Read the model definition and answer for the solid it produces. Units are mm, in the model's axes. Face numbers are marked on the shaded views. A direction names the side the tool comes from. Round coordinates to 2 decimals unless told otherwise and drop trailing zeros. Loops run counter-clockwise (first coordinate to the right, second up) from the corner with the lowest first, then second, coordinate; pieces in that order, holes last. Notation, with made-up numbers: (12.5, 52) - (69.5, 52) arc R21 ccw to (69.5, 80) - close; hole circle Ø10 at (-35.75, 87.25). An arc over 180 degrees is marked (long way). Answer as CSV lines item,"result".
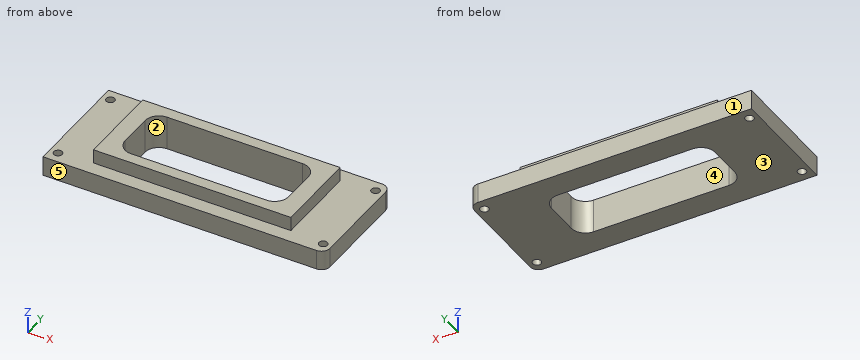
Solid Edge part; units mm, degrees
sketch "Sketch1" plane through (0, 0, 0) normal (0, 0, 1) x (1, 0, 0)
  line L0 (13.4496, 3.5507) -> (113.4496, 3.5507)
  line L1 (113.4496, 3.5507) -> (113.4496, 43.5507)
  line L2 (113.4496, 43.5507) -> (13.4496, 43.5507)
  line L3 (13.4496, 43.5507) -> (13.4496, 3.5507)
extrude "Protrusion1" add sketch "Sketch1" along normal blind 7
hole "Hole_1" at (16.4496, 39.5507, 7) direction (0, 0, -1) diameter 3 end through all
hole "Hole1" at (16.4496, 7.5507, 7) direction (0, 0, -1) diameter 3 end through all
hole "Hole2" at (110.4496, 7.5507, 7) direction (0, 0, -1) diameter 3 end through all
hole "Hole3" at (110.4496, 39.5507, 7) direction (0, 0, -1) diameter 3 end through all
sketch "Sketch2" plane through (63.4496, 23.5507, 7) normal (0, 0, 1) x (1, 0, 0)
  line L0 (-35, 15) -> (35, 15)
  line L1 (35, 15) -> (35, -15)
  line L2 (35, -15) -> (-35, -15)
  line L3 (-35, -15) -> (-35, 15)
extrude "ExtrudedProtrusion_2" add sketch "Sketch2" along normal blind 5
sketch "Sketch3" plane through (63.4496, 23.5507, 12) normal (0, 0, 1) x (0, 1, 0)
  line L0 (-11, -29) -> (11, -29)
  line L1 (11, -29) -> (11, 29)
  line L2 (11, 29) -> (-11, 29)
  line L3 (-11, 29) -> (-11, -29)
  dimension "D1" = 11
  dimension "D2" = 11
extrude "Cutout1" cut sketch "Sketch3" against normal through all
fillet "Round_2" radius 5 4 edges at (34.4496, 34.5507, 6) (34.4496, 12.5507, 6) (92.4496, 12.5507, 6) (92.4496, 34.5507, 6)
fillet "Round_4" radius 3 2 edges at (113.4496, 43.5507, 3.5) (113.4496, 3.5507, 3.5)
1) A cutting plane is placed at B-B, the plane x = 79. Determine the outline of the cut face in (y, z).
Entries:
outline,"(3.55, 0) - (12.55, 0) - (12.55, 12) - (8.55, 12) - (8.55, 7) - (3.55, 7) - close; (34.55, 0) - (43.55, 0) - (43.55, 7) - (38.55, 7) - (38.55, 12) - (34.55, 12) - close"
2) A cutting plane is placed at A-A, the plane y = 22. Determine the outline of the cut face in (x, z), plus the area to 3 significant figures.
Entries:
outline,"(13.45, 0) - (34.45, 0) - (34.45, 12) - (28.45, 12) - (28.45, 7) - (13.45, 7) - close; (92.45, 0) - (113.45, 0) - (113.45, 7) - (98.45, 7) - (98.45, 12) - (92.45, 12) - close"
area,"354 mm^2"
3) The mould has two halves that part along Y. Classify the marked faces 1, 2 and 3: pulls with the +Y half, pulls with the -Y half, needs draft (parallel to the pull), parting line crosses it, or undercut.
Entries:
face 1,"pulls with the +Y half"
face 2,"undercut"
face 3,"needs draft"
4) A cutting plane is placed at C-C, the plane z = 11. Determine the outline of the cut face in (x, y).
Entries:
outline,"(28.45, 8.55) - (98.45, 8.55) - (98.45, 38.55) - (28.45, 38.55) - close; hole (34.45, 17.55) arc R5 ccw to (39.45, 12.55) - (87.45, 12.55) arc R5 ccw to (92.45, 17.55) - (92.45, 29.55) arc R5 ccw to (87.45, 34.55) - (39.45, 34.55) arc R5 ccw to (34.45, 29.55) - close"
5) A cutting plane is placed at D-D, the plane x = 97. Determine the outline of the cut face in (y, z), plus the area to 3 significant figures.
Entries:
outline,"(3.55, 0) - (43.55, 0) - (43.55, 7) - (38.55, 7) - (38.55, 12) - (8.55, 12) - (8.55, 7) - (3.55, 7) - close"
area,"430 mm^2"
6) A tool of negligible diameter and unlimited length cuts with its end or side. For the marked faces 4 and 5, from which of +Z, -Z, +X, -X, +Y, -Y can it reach the whole face along a straight path? Write none if from no direction.
Entries:
face 4,"+Z, -Z"
face 5,"+Z, -Z, +X, -X, -Y"
7) Each of these flat-tipped pins is pushed along its axis until it touches: P1, Ø1.5, axis at x = 72.5, z = 8.5, coming from the -Y side; P2, Ø4, axis at x = 110.45, y = 7.55, coming from the -Z side; P3, Ø1.5, axis at y = 18.5, z = 10.5, coming from the +X side; P4, Ø2, axis at x = 99.5, y = 9, coming from the +Z side. Where does it stop, or does it pass through?
Entries:
P1,"stops at y = 8.55"
P2,"stops at z = 0"
P3,"stops at x = 98.45"
P4,"stops at z = 7"
8) Find the intervals of material crossed by line 1 (X direction, y = 40.5, z = 5.25); line 2 (Y direction, x = 39, z = 9.75); line 3 (Y direction, x = 46, z = 2.25), in increasing order.
Entries:
line 1,"x = 13.45 to 15.29, 17.61 to 109.29, 111.61 to 113.45"
line 2,"y = 8.55 to 12.57, 34.53 to 38.55"
line 3,"y = 3.55 to 12.55, 34.55 to 43.55"
